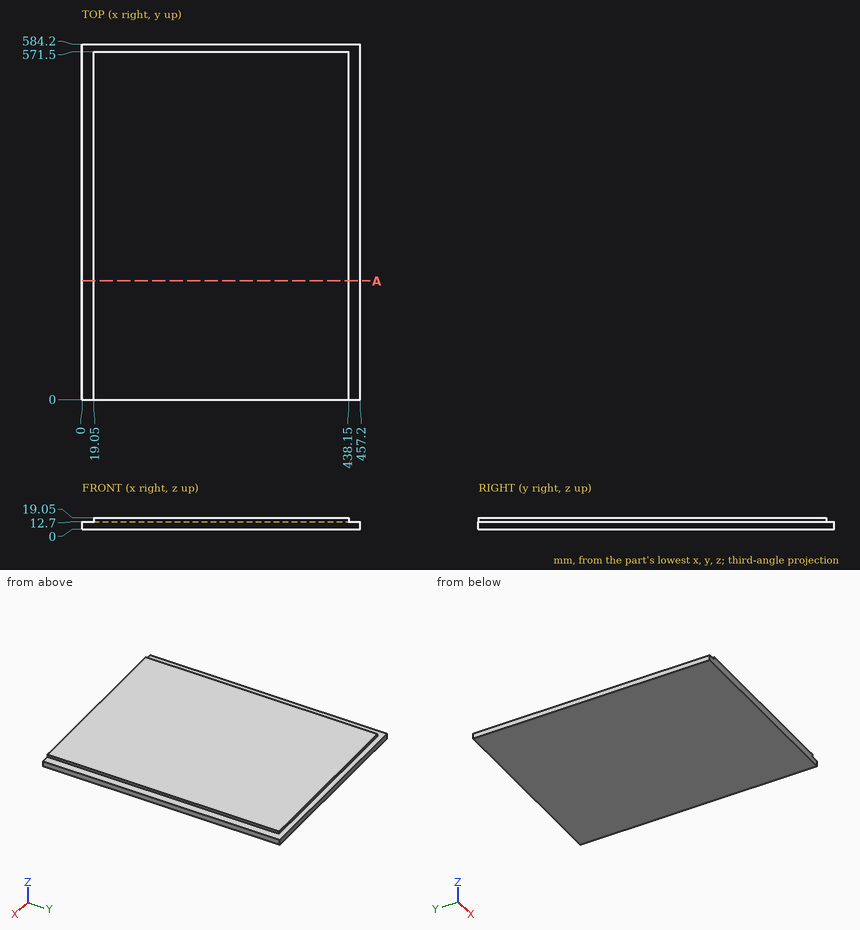
Geometry check sheet. Reference: drawing and pictorial views, mm from the part's lowest x, y, z. Give positions to 0.01 mm unless a question says otherwise; leave off trailing zeros. Write each loop counter-clockwise with the first axis right and the second up, starting at its lowest first coordinate (ties: lowest second). Pieces come first, ordered by that corner, then holes. Notation, with made-up numbers: M 34,57.25 L 60,57.25 A25 cw 60,85.25 Z; hole C 43,-11 d10. An arc over 180 degrees is marked long. Use CSV: the item, a comma, the result in double quotes.
1) Material ranges on line 1 along X through (y, z) = (552, 13); line 2 along Y through (x, z) = (335, 16), recorded low to high.
Final values:
line 1,"19.05 to 438.15"
line 2,"0 to 571.5"
2) Cross-section at A-A (y = 195). Enter the section's corners in (x, z), plus the area to 3 significant figures.
Final values:
outline,"M 0,0 L 457.2,0 L 457.2,12.7 L 438.15,12.7 L 438.15,19.05 L 19.05,19.05 L 19.05,12.7 L 0,12.7 Z"
area,"8,470 mm²"
3) Go/stop test with flat-tipped pins: pin 1 Ø3 at (y, z) = (187, 16) entering from +X; pin 2 Ø4 at (x, z) = (367, 15) entering from +Y; pin 3 Ø3 at (y, z) = (370.5, 15) entering from -X. Record where each tip stops, or that it passes through.
Final values:
pin 1,"x = 438.15"
pin 2,"y = 571.5"
pin 3,"x = 19.05"
